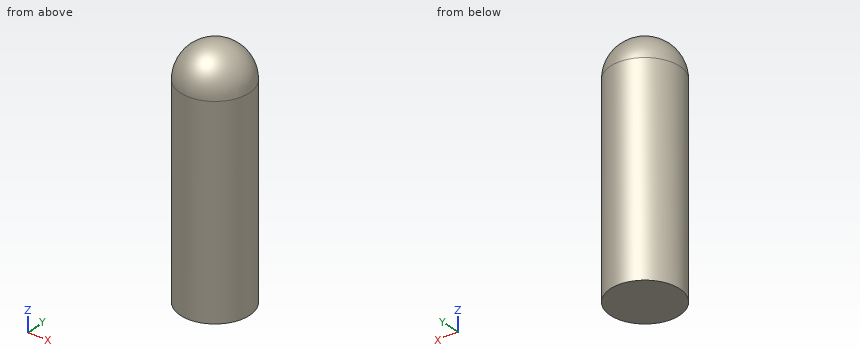
from build123d import *

# Parameters (mm, degrees)
F0_R     = 187.5
F1_DEPTH = 1102.5
F4_R     = 180.5
F5_DEPTH = 1102.5
F6_R     = 187.5
F6_R_2   = 180.5
F7_DEPTH = 5


with BuildPart() as f1:
    # F0 (on Top) → F1 (new body)
    with BuildSketch(Plane.XY):
        Circle(F0_R)
    extrude(amount=F1_DEPTH)

    # F2 (on face) → F3 (revolve)
    with BuildSketch(Plane.XY.offset(1102.5)):
        with BuildLine():
            Line((0, 180.5), (0, 187.5))
            ThreePointArc((0, 187.5), (-187.5, 0), (0, -187.5))
            Line((0, -187.5), (0, -180.5))
            ThreePointArc((0, -180.5), (-180.5, 0), (0, 180.5))
        make_face()
    revolve(axis=Axis((0, -93.75, 1102.5), (0, -1, 0)))

    # F4 (on face) → F5 (cut)
    with BuildSketch(Plane(origin=(0, 0, 0), x_dir=(1, 0, 0), z_dir=(0, 0, -1))):
        Circle(F4_R)
    extrude(amount=-F5_DEPTH, mode=Mode.SUBTRACT)

    # F6 (on face) → F7 (join)
    with BuildSketch(Plane(origin=(0, 0, 0), x_dir=(1, 0, 0), z_dir=(0, 0, -1))):
        Circle(F6_R)
        Circle(F6_R_2)
    extrude(amount=F7_DEPTH)


solid = f1.part
Verification items for the finished model (mm, model axes). Coordinates: 2 decimals unless noted, no trailing zeros. Loops run counter-clockwise (first coordinate to the right, second up) from the corner with the lowest first, then second, coordinate; pieces in that order, holes last. Notation, with made-up numbers: (-22.75, -30.75) -> (5.25, -30.75) arc R15 ccw to (5.25, -24.75) -> close; hole circle Ø9 at (70, -0.5). An arc over 180 degrees is marked (long way). Answer as a JSON object with one key per item and string values. Group by question number.
Item 1: Depth check by flat-ended pin: pin 1 (2 mm diameter, centred on x = -80.5, y = 0.5, fed in from +Z); pin 2 (6 mm diameter, centred on x = 148.5, z = 838, fed in from -Y); pin 3 (3 mm diameter, centred on y = -53.5, z = 1009, fed in from -X). Enter the tip coordinate at first touch or a pass-through.
Item 2: Scan lines: probe 1 along Y at (x, z) = (0, 471); probe 2 along X at (y, z) = (-132, 411). Record each from-to range of solid material in increasing order.
Item 3: Sectioned sample at A-A on x = 0. Record the boundary of the cut face in (y, z).
Item 4: Sectioned sample at C-C on z = 631. Record the boundary of the cut face in (x, y).
Evaluation:
{
 "1": {"pin 1": "stops at z = 1272.31", "pin 2": "stops at y = -118.26", "pin 3": "stops at x = -180.15"},
 "2": {"probe 1": "y = -187.5 to -180.5, 180.5 to 187.5", "probe 2": "x = -133.16 to -123.11, 123.11 to 133.16"},
 "3": {"outline": "(-187.5, -5) -> (187.5, -5) -> (187.5, 1102.5) arc R187.5 ccw to (-187.5, 1102.5) -> close; hole (-180.5, 0) -> (180.5, 0) -> (180.5, 1102.5) arc R180.5 ccw to (-180.5, 1102.5) -> close"},
 "4": {"outline": "circle Ø375 at (0, 0); hole circle Ø361 at (0, 0)"}
}
